Read the model definition and answer for the solid it produces. Units are mm, in the model's axes. Face numbers are marked on the shaded views. A direction names the side the tool comes from. Coordinates: 2 decimals unless noted, no trailing zeros. Order: outer loops, then holes, each group sorted by start corner. A loop starts at its lowest first (then second) coordinate and runs counter-clockwise, first axis right, second up. Notation, with made-up numbers: M -9.75,-19.5 L -5.75,-19.5 A23 ccw -5.75,14.5 Z; hole C 51.5,-16.75 d6. An arc over 180 degrees is marked long. Use a Markdown table: item, result. Add a question column.
1) Find section D-D on x = -10.5. Count the separate pieces of the cut face and the enclosed holes in it, plus the area to 3 significant figures.
2) Find the intervals of material crossed by probe 1 along X at (y, z) = (2.25, 4.5); probe 2 along Z at (x, y) = (10.5, -3.25); probe 3 along X at (y, z) = (1.75, 2.25), in increasing order. Write a range as [from, to].
3) The mould has two halves that part along X. Classify the marked faces 5, 6 and 7: released by +X, released by -X, zero draft, split by the parting line, or undercut.
4) For the marked faces 1, 2, 3 and 4, determine the directions among +Z, -Z, +X, -X, +Y, -Y from which every point of the face is accessible in a straight line to the end or side of a thin tool.
5) Each of these flat-tipped pins is pushed along its axis until it touches: pin 1 Ø1 at (x, z) = (28, 1.5) entering from +Y (3 decimals); pin 2 Ø2 at (x, z) = (-10.5, 4) entering from +Y (3 decimals); pin 3 Ø4.5 at (y, z) = (-1, 7) entering from -X. Where does it stop, or does it pass through?
6) Find section B-B on x = -4.5. Write down the section's boundary in (y, z) (3 decimals), plus the area to 3 significant figures.
7) Find section A-A on y = 0. Write down the section's boundary in (x, z), plus the area to 3 significant figures.
8) Find section C-C on y = 3. Write down the section's boundary in (x, z).
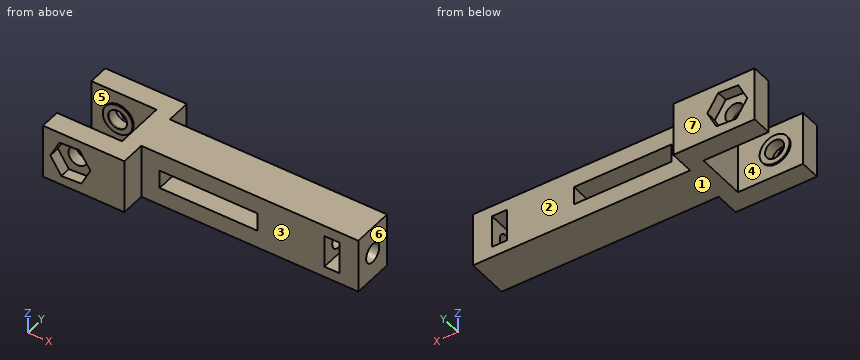
from build123d import *

# Parameters (mm, degrees)
F0_W      = 40
F0_H      = 3.825
F1_DEPTH  = 10
F2_R      = 1.75
F3_DEPTH  = 16.651
F4_W      = 18
F4_H      = 3.4
F4_W_2    = 2.75
F4_H_2    = 6
F5_DEPTH  = 12.151
F6_R      = 1.75
F7_DEPTH  = 15
F10_DEPTH = 2
F11_W     = 17.65
F11_H     = 60
F12_DEPTH = 8
F13_R     = 1.75
F14_DEPTH = 70.001
F15_R     = 2.75
F15_R_2   = 1.75
F16_DEPTH = 0.3
F17_R     = 1.75
F18_DEPTH = 2
F19_R     = 3.75
F20_DEPTH = 1


# Not quite as in the source:
# - a pattern or mirror of a feature is missing from the dataset's text; its kind, count and spacing are read off the source's solid


with BuildPart() as f1:
    # F0 (on Top) → F1 (new body)
    with BuildSketch(Plane.XY):
        Polygon((0, -3.825), (0, 0), (-3, 0), (-3, -4.6), (-15, -4.6), (-15, -8.325), (0, -8.325), align=None)
        Polygon((-3, 0), (0, 0), (0, 3.825), (0, 8.325), (-15, 8.325), (-15, 4.6), (-3, 4.6), align=None)
        with Locations((20, 1.9125)):
            Rectangle(F0_W, F0_H)
        with Locations((20, -1.9125)):
            Rectangle(F0_W, F0_H)
    extrude(amount=F1_DEPTH)

    # F2 (on face) → F3 (cut, through all)
    with BuildSketch(Plane.XZ.offset(8.325)):
        with Locations((-9.9527407438, 5)):
            Circle(F2_R)
    extrude(amount=-F3_DEPTH, mode=Mode.SUBTRACT)

    # F4 (on face) → F5 (cut, through all)
    with BuildSketch(Plane.XZ.offset(3.825)):
        with Locations((12.4002694301, 5)):
            Rectangle(F4_W, F4_H)
        with Locations((35.125, 5)):
            Rectangle(F4_W_2, F4_H_2)
    extrude(amount=-F5_DEPTH, mode=Mode.SUBTRACT)

    # F6 (on face) → F7 (cut)
    with BuildSketch(Plane.YZ.offset(40)):
        with Locations((0, 5)):
            Circle(F6_R)
    extrude(amount=-F7_DEPTH, mode=Mode.SUBTRACT)

    # F15 (on face) → F16 (join)
    with BuildSketch(Plane.XZ.offset(-4.6)):
        with Locations((-9.9527407438, 5)):
            Circle(F15_R)
        with Locations((-9.9527407438, 5)):
            Circle(F15_R_2, mode=Mode.SUBTRACT)
    f16 = extrude(amount=F16_DEPTH)

    # F16_copies: F16 across plane
    add(f16.mirror(Plane(origin=(0, 0, 0), x_dir=(0, 0, -1), z_dir=(0, -1, 0))))

    # F17 (on face) → F18 (cut)
    with BuildSketch(Plane.XZ.offset(8.325)):
        Polygon((-7.9284293953, 1.9088033227), (-6.2635302189, 5.2075067143), (-8.2878415673, 8.2987033916), (-11.9770520922, 8.0911966773), (-13.6419512686, 4.7924932857), (-11.6176399202, 1.7012966084), align=None)
        with Locations((-9.9527407438, 5)):
            Circle(F17_R, mode=Mode.SUBTRACT)
    f18 = extrude(amount=-F18_DEPTH, mode=Mode.SUBTRACT)

    # F18_copies: F18 across plane
    add(f18.mirror(Plane.ZX), mode=Mode.SUBTRACT)


with BuildPart() as f10:
    # F9 (on offset) → F10 (new body)
    with BuildSketch(Plane.YZ.offset(45)):
        Polygon((3.825, 0), (3.825, 10), (3.825, 19.8484882712), (-3.825, 19.8484882712), (-3.825, 10), (-3.825, 0), (-3.825, -10.1515117288), (3.825, -10.1515117288), align=None)
    extrude(amount=F10_DEPTH)

    # F11 (on face) → F12 (join)
    with BuildSketch(Plane.YZ.offset(47)):
        with Locations((0, 4.8484882712)):
            Rectangle(F11_W, F11_H)
    extrude(amount=F12_DEPTH)

    # F13 (on face) → F14 (cut, through all)
    with BuildSketch(Plane.YZ.offset(55)):
        with Locations((0, 5)):
            Circle(F13_R)
    extrude(amount=-F14_DEPTH, mode=Mode.SUBTRACT)

    # F19 (on face) → F20 (join)
    with BuildSketch(Plane(origin=(47, 0, 0), x_dir=(0, -1, 0), z_dir=(-1, 0, 0))):
        with Locations((0, -18)):
            Circle(F19_R)
        with Locations((0, 28)):
            Circle(F19_R)
    extrude(amount=F20_DEPTH)


solid = f1.part
Check result:
| question | item | result |
|---|---|---|
| 1 | separate pieces | 4 |
| 1 | enclosed holes | 0 |
| 1 | area | 38.6 mm2 |
| 2 | probe 1 | x = [-3, 3.4], [21.4, 33.75], [36.5, 40] |
| 2 | probe 2 | z = [0, 3.3], [6.7, 10] |
| 2 | probe 3 | x = [-3, 33.75], [36.5, 40] |
| 3 | face 5 | undercut |
| 3 | face 6 | released by +X |
| 3 | face 7 | zero draft |
| 4 | face 1 | -Z, +X, -X, +Y, -Y |
| 4 | face 2 | +Z, -Z, +X, +Y |
| 4 | face 3 | +Z, -Z, +X, -Y |
| 4 | face 4 | none |
| 5 | pin 1 | stops at y = 3.825 |
| 5 | pin 2 | stops at y = 6.325 |
| 5 | pin 3 | stops at x = -3 |
| 6 | outline | M -8.325,0 L -4.6,0 L -4.6,10 L -8.325,10 Z; M 4.6,0 L 8.325,0 L 8.325,10 L 4.6,10 Z |
| 6 | area | 74.5 mm2 |
| 7 | outline | M -3,0 L 40,0 L 40,3.25 L 36.5,3.25 L 36.5,2 L 33.75,2 L 33.75,3.25 L 25,3.25 L 25,6.75 L 33.75,6.75 L 33.75,8 L 36.5,8 L 36.5,6.75 L 40,6.75 L 40,10 L -3,10 Z; hole M 3.4,3.3 L 21.4,3.3 L 21.4,6.7 L 3.4,6.7 Z |
| 7 | area | 309 mm2 |
| 8 | outline | M -3,0 L 40,0 L 40,10 L -3,10 Z; hole M 3.4,3.3 L 21.4,3.3 L 21.4,6.7 L 3.4,6.7 Z; hole M 33.75,2 L 36.5,2 L 36.5,8 L 33.75,8 Z |
